Input: part model. Units: mm. Frame: model coordinates. A direction names the side the tool comes from. Round coordinates to 2 decimals unless told otherwise and drop trailing zeros. Loops run counter-clockwise (first coordinate to the right, second up) from the corner with the lowest first, then second, coordinate; pieces in that order, holes last. Notation, with made-up numbers: M 8,-19 L 47,-19 A21 cw 47,9 Z; hole C -10.5,20.25 d7. An arc over 180 degrees is marked long. Return JSON: item names as keys, results as strings. Group by question number.
1) Mould query, pull axis Z, two halves, no side actions, for faces 1 (the face through (25.4, -6, -9)), 2 (the face through (-0.356, 7.559, -5.796)), 3 (the face through (0.04, 7.83, -13.81)). Classes: +Z half, -Z half, draft (parallel to the pull), parting line (faces both ways), or undercut.
2) Material intervals for line 1 (Z direction, x = 8, y = -0.5); line 2 (Y direction, x = -21, z = -6); line 3 (X direction, y = -13, z = -10.5) (3 decimals), sorted ascending. Write a range as from..to.
3) Access query for faces 4 (the face through (0.044, 8.049, 13.684)), 5 (the face through (14.132, 4.005, -12.719)), 6 (the face through (-3.175, -11, -8)). Directions: +Z, -Z, +X, -X, +Y, -Y. A direction counts if a zero-diameter tool reaches every point of the face in a straight line with its end or side. Return the directions, or none.
4) Contact query for flat-ended pins moving along their axis: P1, Ø1, axis at x = 8.5, z = -11.5, coming from the +Y side; P2, Ø10, axis at x = -17, z = -1, coming from the +Y side (3 decimals); P3, Ø4, axis at y = -2, z = 6.5, coming from the +X side; P4, Ø2, axis at x = -19.5, y = 8, coming from the -Z side. Output: stop coordinate, or through.
5) Section A-A (z = 0). Output: boundary loops of the cut face in (x, y) (3 decimals).
6) Section C-C (x = 7). Output: boundary loops of the cut face in (y, z) (3 decimals).
7) Section B-B (y = 7). Output: boundary loops of the cut face in (x, z) (3 decimals), plus the area to 3 significant figures.
8) Section D-D (z = -11). Output: boundary loops of the cut face in (x, y) (3 decimals).
from build123d import *

# Parameters (mm, degrees)
PAD_DEPTH            = 3.175
CYLINDER_R           = 13.335
CYLINDER_DEPTH       = 50.8
CYLINDER_PITCH_ANGLE = 90
SKETCH002_R          = 9.525
POCKET_DEPTH         = 50.801


with BuildPart() as pad:
    # Sketch001 → Pad (new body, symmetric)
    with BuildSketch(Plane.YZ):
        Polygon((15.875, 9.165436), (0, 18.330871), (-15.875, 9.165436), (-15.875, -9.165436), (0, -18.330871), (15.875, -9.165436), align=None)
    extrude(amount=PAD_DEPTH, both=True)


with BuildPart() as pocket:
    # Cylinder → Cylinder (new body)
    with BuildSketch(Plane.XY):
        Circle(CYLINDER_R)
    extrude(amount=CYLINDER_DEPTH)


with BuildPart() as pocket_1:
    # Cylinder pitch: moved
    add(pocket.part.rotate(Axis((0, 0, 0), (0, 1, 0)), CYLINDER_PITCH_ANGLE))


with BuildPart() as pocket_2:
    # Cylinder placement: moved
    add(pocket_1.part.moved(Location((-25.4, 0, 0))))

    # Fusion: union Pad
    add(pad.part)

    # Sketch002 → Pocket (cut, through all)
    with BuildSketch(Plane(origin=(-25.4, 0, 0), x_dir=(0, -1, 0), z_dir=(-1, 0, 0))):
        Circle(SKETCH002_R)
    extrude(amount=-POCKET_DEPTH, mode=Mode.SUBTRACT)


solid = pocket_2.part
Returned:
{
 "1": {"face 1": "draft", "face 2": "undercut", "face 3": "-Z half"},
 "2": {"line 1": "z = -13.33..-9.51, 9.51..13.33", "line 2": "y = -11.91..-7.4, 7.4..11.91", "line 3": "x = -3.175..3.175"},
 "3": {"face 4": "+Z, +X, -X, +Y", "face 5": "+X", "face 6": "-X"},
 "4": {"P1": "stops at y = 7.54", "P2": "stops at y = 13.335", "P3": "passes through", "P4": "stops at z = -11.35"},
 "5": {"outline": "M -25.4,-13.335 L -3.175,-13.335 L -3.175,-15.875 L 3.175,-15.875 L 3.175,-13.335 L 25.4,-13.335 L 25.4,-9.525 L -25.4,-9.525 Z; M -25.4,9.525 L 25.4,9.525 L 25.4,13.335 L 3.175,13.335 L 3.175,15.875 L -3.175,15.875 L -3.175,13.335 L -25.4,13.335 Z"},
 "6": {"outline": "C 0,0 d26.67; hole C 0,0 d19.05"},
 "7": {"outline": "M -25.4,-11.35 L -3.175,-11.35 L -3.175,-14.289 L 3.175,-14.289 L 3.175,-11.35 L 25.4,-11.35 L 25.4,-6.46 L -25.4,-6.46 Z; M -25.4,6.46 L 25.4,6.46 L 25.4,11.35 L 3.175,11.35 L 3.175,14.289 L -3.175,14.289 L -3.175,11.35 L -25.4,11.35 Z", "area": "534 mm^2"},
 "8": {"outline": "M -25.4,-7.538 L -3.175,-7.538 L -3.175,-12.697 L 3.175,-12.697 L 3.175,-7.538 L 25.4,-7.538 L 25.4,7.538 L 3.175,7.538 L 3.175,12.697 L -3.175,12.697 L -3.175,7.538 L -25.4,7.538 Z"}
}
